from build123d import *

# Parameters (mm, degrees)
EXTRUDE_1_DEPTH = 3


with BuildPart() as part:
    # Эскиз2 → Бобышка-Вытянуть1 (new body)
    with BuildSketch(Plane.XY):
        with BuildLine():
            Line((0, 0), (244, 0))
            Line((244, 0), (244, 6))
            Line((244, 6), (250, 6))
            Line((250, 6), (250, 12))
            Line((250, 12), (244, 12))
            Line((244, 12), (214, 12))
            Line((214, 12), (214, 20))
            Line((214, 20), (187, 20))
            Line((187, 20), (187, 32))
            ThreePointArc((187, 32), (196.668498224, 58.076809621), (221, 71.547439867))
            Line((221, 71.547439867), (231, 71.547439867))
            Line((231, 71.547439867), (231, 51.547439867))
            Line((231, 51.547439867), (241, 51.547439867))
            Line((241, 51.547439867), (241, 83.547439867))
            ThreePointArc((241, 83.547439867), (238.656854249, 89.204294116), (233, 91.547439867))
            Line((233, 91.547439867), (219.644566271, 91.547439867))
            ThreePointArc((219.644566271, 91.547439867), (182.048214587, 71.740873017), (167, 32))
            Line((167, 32), (167, 20))
            Line((167, 20), (0, 20))
            Line((0, 20), (-6, 20))
            Line((-6, 20), (-6, 14))
            Line((-6, 14), (0, 14))
            Line((0, 14), (0, 6))
            Line((0, 6), (-6, 6))
            Line((-6, 6), (-6, 0))
            Line((-6, 0), (0, 0))
        make_face()
    extrude(amount=EXTRUDE_1_DEPTH)


solid = part.part
Verification items for the finished model (mm, model axes). Give positions to 0.01 mm unless a question says otherwise; leave off trailing zeros. Write each loop counter-clockwise with the first axis right and the second up, starting at its lowest first coordinate (ties: lowest second). Pieces come first, ordered by that corner, then holes.
(1) Mould release check, pull along X, two halves, no side actions. Record for faces 1 (the face through (140, 15, 0)), 2 (the face through (196.41, 57.77, 1.48)), 3 (the face through (182.45, 72.19, 1.48)): +X half, -X half, draft (parallel to the pull), parting line (faces both ways), or undercut.
(2) Cross-section at B-B (y = 28). Enter the section's corners in (x, z), plus the area to 3 significant figures.
(3) Material ranges on line 1 (Y direction, x = 96.5, z = 0.35); line 2 (X direction, y = 59, z = 2.65); line 3 (X direction, y = 67.5, z = 1.65), recorded low to high.
(4) Gauge pin test, flat ends, axial feed: pin 1 (0.9 mm diameter, centred on x = 199, z = 2, fed in from +Y); pin 2 (1.5 mm diameter, centred on y = 27.5, z = 1, fed in from +X); pin 3 (0.9 mm diameter, centred on x = -4.5, z = 1, fed in from +Y); pin 4 (1.5 mm diameter, centred on x = 204, y = 62, fed in from +Z). Record the tip position at first contact, or that the pin passes through.
(5) Cross-section at A-A (z = 0.6). Enter the section's corners in (x, y).
(6) Cross-section at C-C (x = 94). Enter the section's corners in (y, z), plus the area to 3 significant figures.
Worked out:
1. face 1: draft
1. face 2: undercut
1. face 3: -X half
2. outline: (167, 0) - (187, 0) - (187, 3) - (167, 3) - close
2. area: 60.0 mm2
3. line 1: y = 0 to 20
3. line 2: x = 173.42 to 197.49, 231 to 241
3. line 3: x = 178.63 to 208.57, 231 to 241
4. pin 1: stops at y = 85.3
4. pin 2: stops at x = 187
4. pin 3: stops at y = 20
4. pin 4: passes through
5. outline: (-6, 0) - (244, 0) - (244, 6) - (250, 6) - (250, 12) - (214, 12) - (214, 20) - (187, 20) - (187, 32) arc R40 cw to (221, 71.55) - (231, 71.55) - (231, 51.55) - (241, 51.55) - (241, 83.55) arc R8 ccw to (233, 91.55) - (219.64, 91.55) arc R60 ccw to (167, 32) - (167, 20) - (-6, 20) - (-6, 14) - (0, 14) - (0, 6) - (-6, 6) - close
6. outline: (0, 0) - (20, 0) - (20, 3) - (0, 3) - close
6. area: 60.0 mm2
